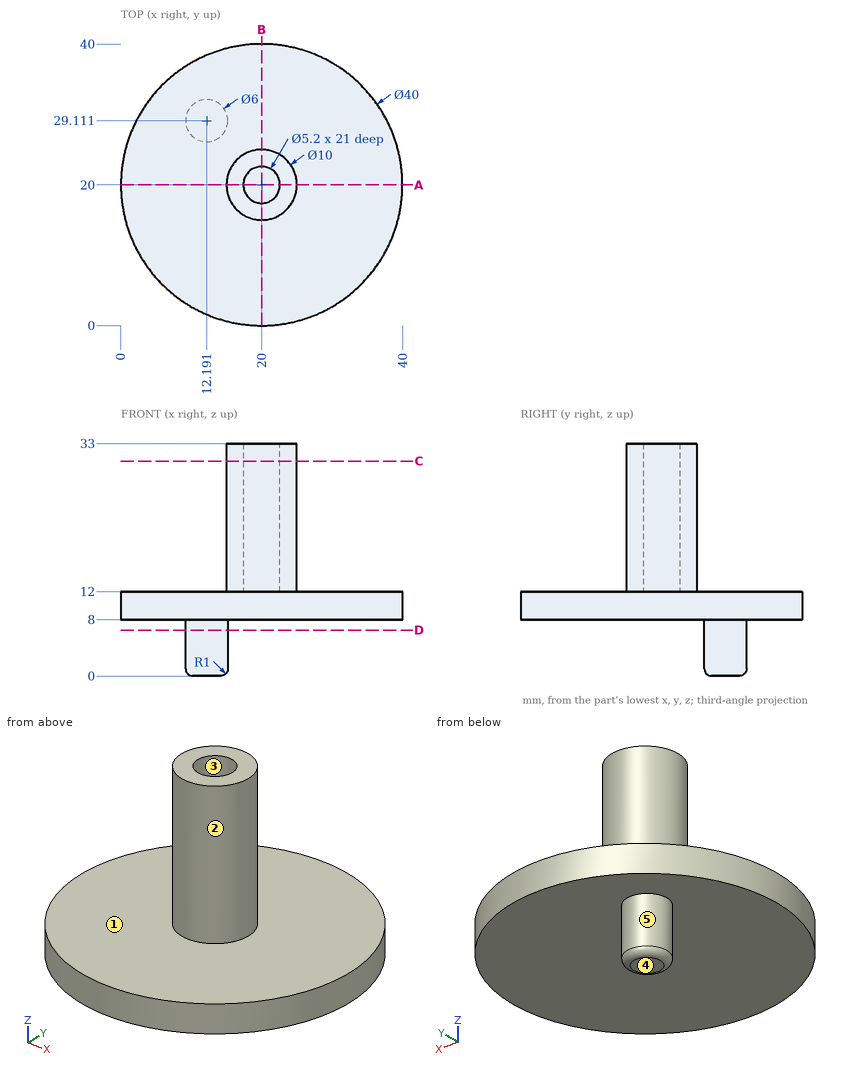
Design review of the part shown in the three views and the two pictorial views. Dimensions are in mm from the part's minimum x, y and z. A direction names the side the tool comes from. Give positions to 0.01 mm unless a question says otherwise; leave off trailing zeros. Loops run counter-clockwise (first coordinate to the right, second up) from the corner with the lowest first, then second, coordinate; pieces in that order, holes last. Notation, with made-up numbers: (-7, -21.5) - (26, -21.5) arc R20 ccw to (26, -0.5) - close; hole circle Ø6 at (18, 28). An arc over 180 degrees is marked (long way). Use CSV: the item, a comma, the result in double quotes. Start each with the question number.
1. Insertion check: P1, Ø7, axis at x = 20, y = 20, coming from the -Z side; P2, Ø1.6, axis at x = 20.5, y = 21, coming from the +Z side; P3, Ø2, axis at x = 24, z = 27.5, coming from the +Y side; P4, Ø12, axis at x = 7, z = 19, coming from the -Y side. Each pin has a flat end and moves straight along its axis. Give the tip position at first contact, or say it passes through.
2. Add section C-C (z = 30.5). State the section outline as (x, y) points.
3. Wall thickness on L1, parallel to Y at x = 20, z = 23; L2, parallel to Z at x = 12.5, y = 23: over which ranges is each line inside the solid? List them lowest first.
4. Machinability: for the marked faces 4 and 5, which of the approach directions +Z, -Z, +X, -X, +Y, -Y give a long, thin tool a straight path to every point of the face, cutting with its end or side? Answer none if there is none.
5. Draft analysis for pull direction X (two halves, no side actions). For the marked faces 1, 2 and 3, state which applies: released by +X, released by -X, zero draft, split by the parting line, or undercut.
6. Add section D-D (z = 6.5). State the section outline as (x, y) points.
7. Add section A-A (y = 20). State the section outline as (x, z) points.
Results found:
1,P1,"stops at z = 8"
1,P2,"stops at z = 12"
1,P3,"stops at y = 24"
1,P4,"passes through"
2,outline,"circle Ø10 at (20, 20); hole circle Ø5.2 at (20, 20)"
3,L1,"y = 15 to 17.4, 22.6 to 25"
3,L2,"z = 8 to 12"
4,face 4,"-Z, +X, -X, +Y, -Y"
4,face 5,"-Z"
5,face 1,"zero draft"
5,face 2,"split by the parting line"
5,face 3,"undercut"
6,outline,"circle Ø6 at (12.19, 29.11)"
7,outline,"(0, 8) - (40, 8) - (40, 12) - (25, 12) - (25, 33) - (22.6, 33) - (22.6, 12) - (17.4, 12) - (17.4, 33) - (15, 33) - (15, 12) - (0, 12) - close"
